Here's the drawing with two shaded views (mm, measured from the low corner). I have some questions. A direction names the side the tool comes from. Give positions to 0.01 mm unless a question says otherwise; leave off trailing zeros. Write each loop counter-clockwise with the first axis right and the second up, starting at its lowest first coordinate (ties: lowest second). Pieces come first, ordered by that corner, then holes. Notation, with made-up numbers: M 23,-4.75 L 48,-4.75 A31 cw 48,33.25 Z; hole C 83.5,87.25 d1. An arc over 180 degrees is marked long. Use one line per item in the form item = value. Start each with the question number.
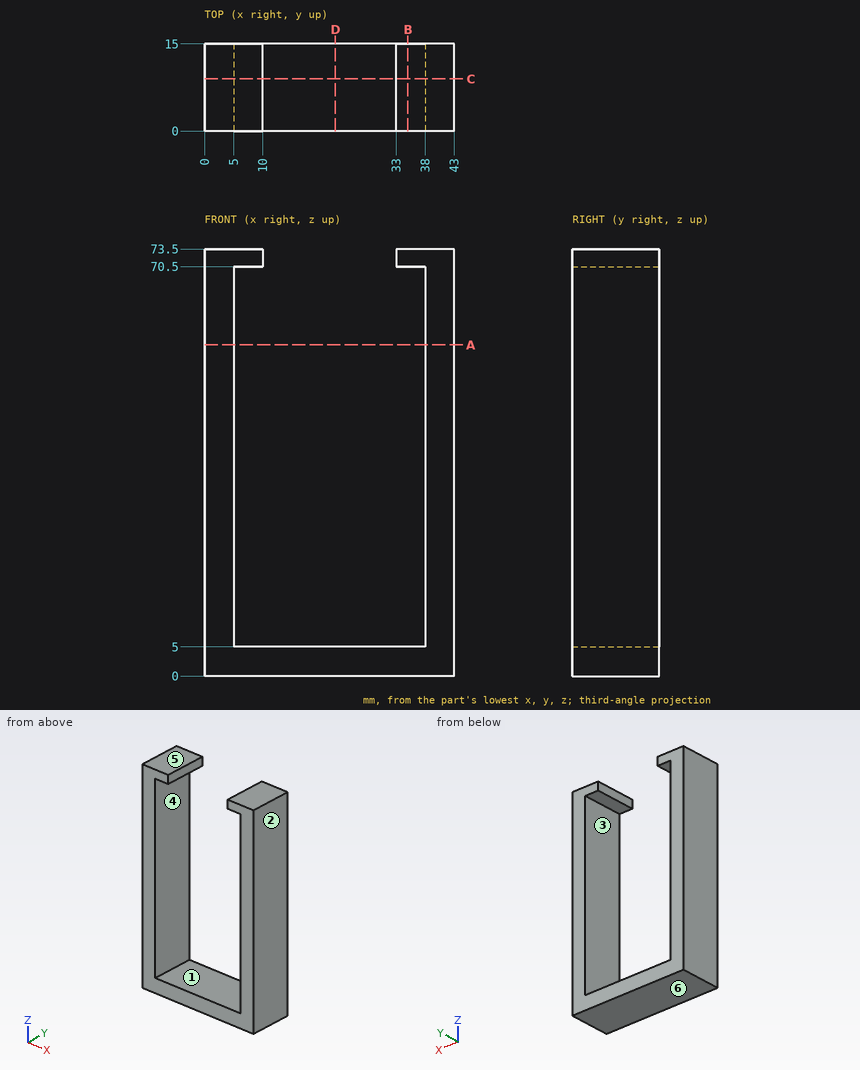
1) Suppose I cut it at B-B, the plane x = 35. List the corners of the cut face in (y, z) for me, and give its area (3 significant figures).
2) Thinking about a two-plate mould opening in Z: for the marked faces 3, 4, 5 and 6, which applies, released by +Z, released by -Z, zero draft, split by the parting line, or undercut?
3) Suppose I cut it at D-D, the plane x = 22.5. List the corners of the cut face in (y, z) for me, and give its area (3 significant figures).
4) On a 3-axis mill with a long thin cutter (end or side, diameter ignored), from which of +Z, -Z, +X, -X, +Y, -Y can I reach the whole of each face in a straight line? I mean the marked faces 1 and 2. Say none if no direction works.
5) Please list where these lines run through material, in increasing order: line 1 (X direction, y = 4, z = 51); line 2 (Z direction, x = 7, y = 0.5); line 3 (Z direction, x = 28, y = 3.25).
6) Suppose I cut it at C-C, the plane y = 9. List the corners of the cut face in (x, z) for me.
7) Suppose I cut it at A-A, the plane z = 57. List the corners of the cut face in (x, y) for me, and give its area (3 significant figures).
8) Will these pins go through, and if not, where does the flat tip stop? P1, Ø5, axis at x = 37, z = 34, coming from the +Y side; P2, Ø4.5, axis at x = 17.5, y = 4, coming from the +Z side; P3, Ø12, axis at x = 29.5, z = 41, coming from the -Y side.
Checks:
q1.outline = M 0,0 L 15,0 L 15,5 L 0,5 Z; M 0,70.5 L 15,70.5 L 15,73.5 L 0,73.5 Z
q1.area = 120 mm^2
q2.face_3 = undercut
q2.face_4 = undercut
q2.face_5 = released by +Z
q2.face_6 = released by -Z
q3.outline = M 0,0 L 15,0 L 15,5 L 0,5 Z
q3.area = 75.0 mm^2
q4.face_1 = +Y, -Y
q4.face_2 = +Z, -Z, +X, +Y, -Y
q5.line_1 = 0 to 5, 38 to 43
q5.line_2 = 0 to 5, 70.5 to 73.5
q5.line_3 = 0 to 5
q6.outline = M 0,0 L 43,0 L 43,73.5 L 33,73.5 L 33,70.5 L 38,70.5 L 38,5 L 5,5 L 5,70.5 L 10,70.5 L 10,73.5 L 0,73.5 Z
q7.outline = M 0,0 L 5,0 L 5,15 L 0,15 Z; M 38,0 L 43,0 L 43,15 L 38,15 Z
q7.area = 150 mm^2
q8.P1 = 15
q8.P2 = 5
q8.P3 = through
